Could you check a few things on this drawing? It's one solid part, dimensions in mm from its lowest x, y, z. A direction names the side the tool comes from. Give positions to 0.01 mm unless a question says otherwise; leave off trailing zeros. Write each loop counter-clockwise with the first axis right and the second up, starting at its lowest first coordinate (ties: lowest second). Pieces come first, ordered by that corner, then holes.
1. If I drill on probe 1 along Z at (x, y) = (69.85, 2) (3 decimals); probe 2 along Z at (x, y) = (38.1, 2); probe 3 along X at (y, z) = (4.25, 44.5), over which ranges is the centre line in solid material (lowest first)?
2. Suppose I cut it at B-B (y = 2.25). Give the number of separate pieces and of enclosed holes in the cut face, and give its area (3 significant figures).
3. Suppose I cut it at A-A (z = 50.5). Please give me the cut outline in (x, y).
4. Suppose I cut it at C-C (x = 33.5). Please give me the cut outline in (y, z), and give its area (3 significant figures).
5. Thinking about a two-plate mould opening in X: for the marked faces 3, 4, 5 and 6, which applies, pulls with the +X half, pulls with the -X half, needs draft (parallel to the pull), parting line crosses it, or undercut?
6. On a 3-axis mill with a long thin cutter (end or side, diameter ignored), from which of +Z, -Z, +X, -X, +Y, -Y can I reach the whole of each face in a straight line? I mean the marked faces 1 and 2. Say none if no direction works.
7. I'm going to push flat-ended pins straight in: pin 1 (4 mm diameter, centred on x = 6.35, z = 12.7, fed in from +Y); pin 2 (1 mm diameter, centred on x = 33, y = 5, fed in from +Z); pin 3 (1.5 mm diameter, centred on y = 1, z = 35.5, fed in from -X); pin 4 (1.5 mm diameter, centred on y = 5, z = 30.5, fed in from -X). Where does each tip first touch, or does it pass through?
8. Suppose I cut it at D-D (x = 13.5). Please give me the cut outline in (y, z).
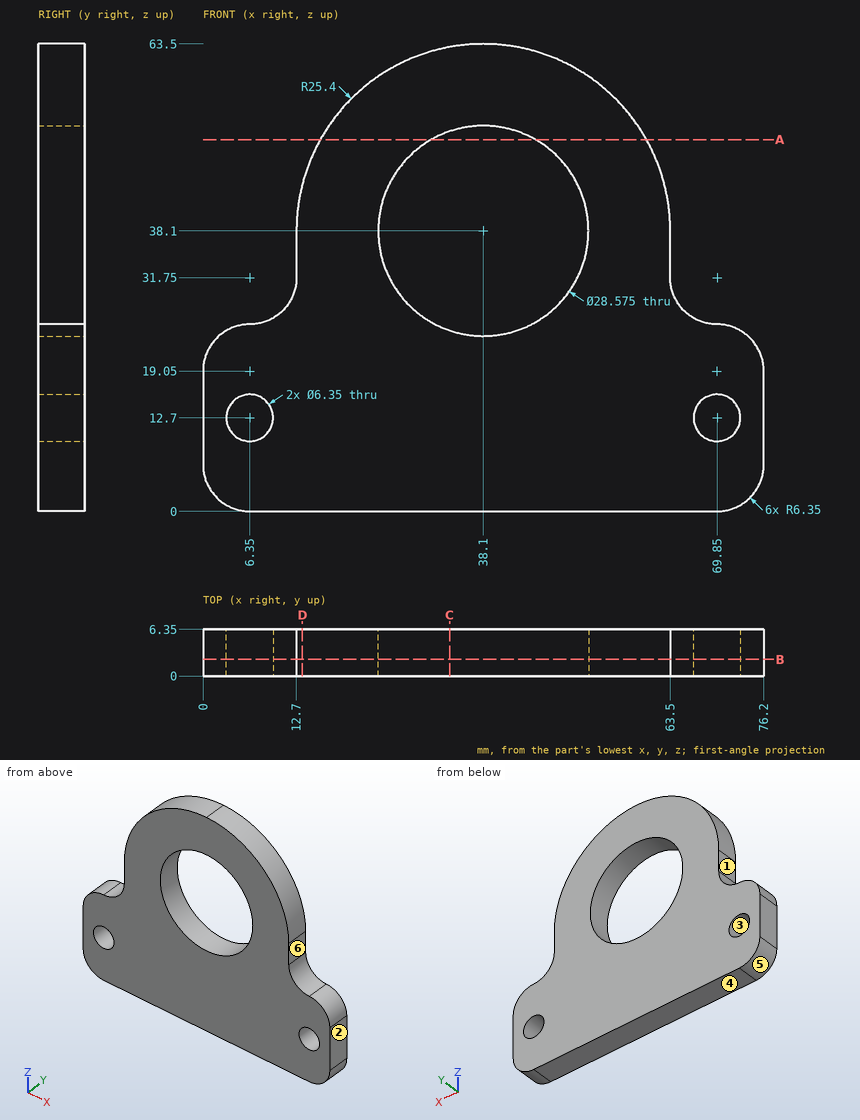
Checks:
1. probe 1: z = 0 to 9.525, 15.875 to 25.4
1. probe 2: z = 0 to 23.81, 52.39 to 63.5
1. probe 3: x = 13.52 to 25.33, 50.87 to 62.68
2. separate pieces: 1
2. enclosed holes: 3
2. area: 2,870 mm2
3. outline: (15.93, 0) - (31, 0) - (31, 6.35) - (15.93, 6.35) - close; (45.2, 0) - (60.27, 0) - (60.27, 6.35) - (45.2, 6.35) - close
4. outline: (0, 0) - (6.35, 0) - (6.35, 24.57) - (0, 24.57) - close; (0, 51.63) - (6.35, 51.63) - (6.35, 63.08) - (0, 63.08) - close
4. area: 229 mm2
5. face 3: undercut
5. face 4: needs draft
5. face 5: pulls with the -X half
5. face 6: pulls with the +X half
6. face 1: +Z, -X, +Y, -Y
6. face 2: +Z, -Z, +X, +Y, -Y
7. pin 1: passes through
7. pin 2: stops at z = 63.08
7. pin 3: stops at x = 12.7
7. pin 4: stops at x = 12.38
8. outline: (0, 0) - (6.35, 0) - (6.35, 44.42) - (0, 44.42) - close
